Design review of the part built by this model. Coordinates are the model's own, in mm. Face numbers are marked on the shaded views. A direction names the side the tool comes from. Coordinates: 2 decimals unless noted, no trailing zeros. Loops run counter-clockwise (first coordinate to the right, second up) from the corner with the lowest first, then second, coordinate; pieces in that order, holes last. Notation, with made-up numbers: (53, 63) -> (105, 63) arc R15 ccw to (105, 81) -> close; hole circle Ø5 at (-9, -15.75). An arc over 180 degrees is marked (long way). One line per item, written item: value. Start each with the question number.
1. Machinability: for the marked faces 1, 2 and 3, which of the approach directions +Z, -Z, +X, -X, +Y, -Y give a long, thin tool a straight path to every point of the face, cutting with its end or side? Answer none if there is none.
2. For probe 1 along Z at (x, y) = (0, 12); probe 2 along X at (y, z) = (-7, -8.25); probe 3 along Z at (x, y) = (8.5, 13.5), list the stretches that pass through material, from the lowest coordinate up.
3. Add section D-D on y = -8.5. Write out the cut boundary in (x, z).
4. Insertion check: pin 1 (3.5 mm diameter, centred on x = -12, z = -2.5, fed in from -Y); pin 2 (5 mm diameter, centred on x = 3, z = -7, fed in from -Y); pin 3 (3 mm diameter, centred on x = -11.5, z = -3.5, fed in from +Y); pin 4 (6 mm diameter, centred on x = 1, z = -2.5, fed in from -Y). Each pin has a flat end and moves straight along its axis. Give the tip position at first contact, or say it passes through.
5. Add section A-A on z = -6.5. Write out the cut boundary in (x, y).
6. Add section B-B on y = 3.5. Write out the cut boundary in (x, z), plus the area to 3 significant figures.
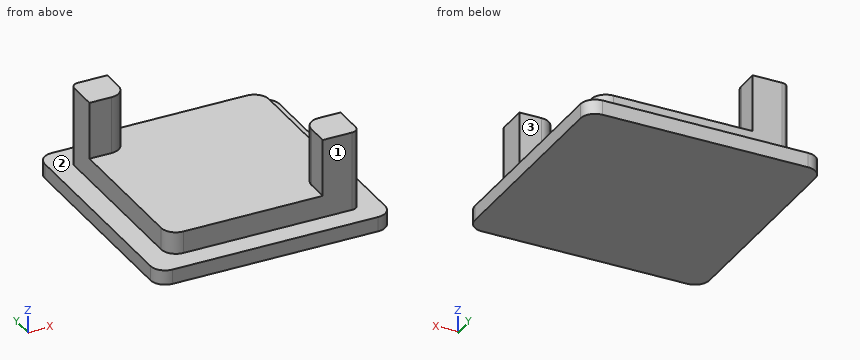
```python
from build123d import *

# Parameters (mm, degrees)
BOX013_W     = 26
BOX013_H     = 26
BOX013_DEPTH = 3
BOX014_W     = 5
BOX014_H     = 5
BOX014_DEPTH = 7.8
BOX015_W     = 5
BOX015_H     = 5
BOX015_DEPTH = 7.8
BOX012_W     = 32
BOX012_H     = 32
BOX012_DEPTH = 2
FILLET_R     = 2
FILLET001_R  = 1
FILLET002_R  = 2


with BuildPart() as obj1:
    # Box013 → Box013 (new body)
    with BuildSketch(Plane(origin=(-13, -13, -10), x_dir=(1, 0, 0), z_dir=(0, 0, 1))):
        with Locations((13, 13)):
            Rectangle(BOX013_W, BOX013_H)
    extrude(amount=BOX013_DEPTH)


with BuildPart() as obj2:
    # Box014 → Box014 (new body)
    with BuildSketch(Plane(origin=(-13, 8, -7), x_dir=(1, 0, 0), z_dir=(0, 0, 1))):
        with Locations((2.5, 2.5)):
            Rectangle(BOX014_W, BOX014_H)
    extrude(amount=BOX014_DEPTH)


with BuildPart() as obj3:
    # Box015 → Box015 (new body)
    with BuildSketch(Plane(origin=(8, -13, -7), x_dir=(1, 0, 0), z_dir=(0, 0, 1))):
        with Locations((2.5, 2.5)):
            Rectangle(BOX015_W, BOX015_H)
    extrude(amount=BOX015_DEPTH)


with BuildPart() as fillet002:
    # Box012 → Box012 (new body)
    with BuildSketch(Plane(origin=(-16, -16, -12), x_dir=(1, 0, 0), z_dir=(0, 0, 1))):
        with Locations((16, 16)):
            Rectangle(BOX012_W, BOX012_H)
    extrude(amount=BOX012_DEPTH)

    # Fusion001: union obj1, obj2, obj3
    add(obj1.part)
    add(obj2.part)
    add(obj3.part)

    # Fillet
    fillet_edges = [fillet002.edges().sort_by_distance(p)[0] for p in [
        (-8, 8, -3.1),
        (8, -8, -3.1),
    ]]
    fillet(fillet_edges, radius=FILLET_R)

    # Fillet001
    fillet001_edges = [fillet002.edges().sort_by_distance(p)[0] for p in [
        (-13, 13, -3.1),
        (13, -13, -3.1),
    ]]
    fillet(fillet001_edges, radius=FILLET001_R)

    # Fillet002
    fillet002_edges = [fillet002.edges().sort_by_distance(p)[0] for p in [
        (-13, -13, -8.5),
        (13, 13, -8.5),
        (-16, -16, -11),
        (-16, 16, -11),
        (16, 16, -11),
        (16, -16, -11),
    ]]
    fillet(fillet002_edges, radius=FILLET002_R)


solid = fillet002.part
```
Worked answers:
1. face 1: +Z, +X, -X, -Y
1. face 2: +Z
1. face 3: +Z, +X, -X, +Y
2. probe 1: z = -12 to -7
2. probe 2: x = -13 to 13
2. probe 3: z = -12 to -10
3. outline: (-16, -12) -> (16, -12) -> (16, -10) -> (13, -10) -> (13, 0.8) -> (8.68, 0.8) -> (8.68, -7) -> (-13, -7) -> (-13, -10) -> (-16, -10) -> close
4. pin 1: stops at y = 8
4. pin 2: stops at y = -13
4. pin 3: stops at y = 13
4. pin 4: passes through
5. outline: (-13, 8) -> (-10, 8) arc R2 ccw to (-8, 10) -> (-8, 13) -> (-12, 13) arc R1 ccw to (-13, 12) -> close; (8, -13) -> (12, -13) arc R1 ccw to (13, -12) -> (13, -8) -> (10, -8) arc R2 ccw to (8, -10) -> close
6. outline: (-16, -12) -> (16, -12) -> (16, -10) -> (13, -10) -> (13, -7) -> (-13, -7) -> (-13, -10) -> (-16, -10) -> close
6. area: 142 mm²
